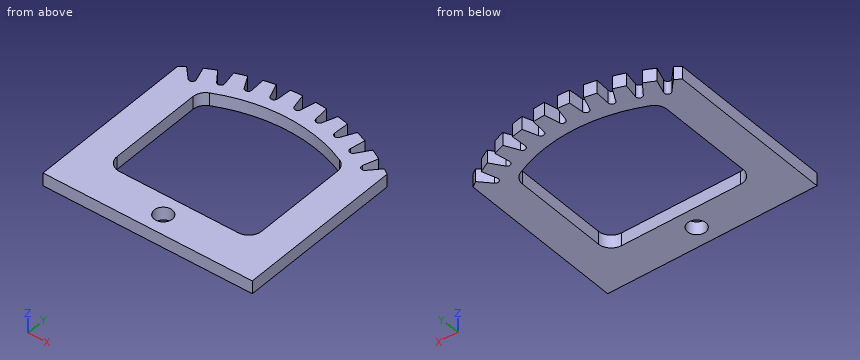
from build123d import *

# Parameters (mm, degrees)
ESQUISSE1_R        = 7
BOSS_EXTRU_2_DEPTH = 5


with BuildPart() as part:
    # Esquisse1 → Boss.-Extru.2 (new body, symmetric)
    with BuildSketch(Plane.XY):
        with BuildLine():
            Line((-81, 114.188440746), (-81, -15))
            Line((-81, -15), (81, -15))
            Line((81, -15), (81, 114.188440746))
            ThreePointArc((81, 114.188440746), (78.796472268, 115.719989449), (76.563994166, 117.209021825))
            Line((76.563994166, 117.209021825), (68.597490223, 108.845387152))
            ThreePointArc((68.597490223, 108.845387152), (65.420366542, 108.419035897), (64.316466092, 111.428569759))
            Line((64.316466092, 111.428569759), (68.001945903, 122.375387041))
            ThreePointArc((68.001945903, 122.375387041), (64.034003077, 124.497576081), (59.999908366, 126.491149872))
            Line((59.999908366, 126.491149872), (53.238382738, 117.126464015))
            ThreePointArc((53.238382738, 117.126464015), (50.148170341, 116.274127452), (48.64719318, 119.10661008))
            Line((48.64719318, 119.10661008), (50.81752925, 130.451442004))
            ThreePointArc((50.81752925, 130.451442004), (46.598920029, 132.017198319), (42.332170661, 133.446571058))
            Line((42.332170661, 133.446571058), (36.899996383, 123.253090169))
            ThreePointArc((36.899996383, 123.253090169), (33.953537336, 121.990446371), (32.083092779, 124.593776437))
            Line((32.083092779, 124.593776437), (32.698363453, 136.127943595))
            ThreePointArc((32.698363453, 136.127943595), (28.306685892, 137.10846631), (23.88576542, 137.947345789))
            Line((23.88576542, 137.947345789), (19.882863135, 127.112571065))
            ThreePointArc((19.882863135, 127.112571065), (17.134355274, 125.462845387), (14.928848702, 127.789136649))
            Line((14.928848702, 127.789136649), (13.977736553, 139.300476958))
            ThreePointArc((13.977736553, 139.300476958), (9.493772162, 139.677730115), (5, 139.910685796))
            Line((5, 139.910685796), (2.5, 128.633914537))
            ThreePointArc((2.5, 128.633914537), (0, 126.627452408), (-2.5, 128.633914537))
            Line((-2.5, 128.633914537), (-5, 139.910685796))
            ThreePointArc((-5, 139.910685796), (-9.493772162, 139.677730115), (-13.977736553, 139.300476958))
            Line((-13.977736553, 139.300476958), (-14.928848702, 127.789136649))
            ThreePointArc((-14.928848702, 127.789136649), (-17.134355274, 125.462845387), (-19.882863135, 127.112571065))
            Line((-19.882863135, 127.112571065), (-23.88576542, 137.947345789))
            ThreePointArc((-23.88576542, 137.947345789), (-28.306685892, 137.10846631), (-32.698363453, 136.127943595))
            Line((-32.698363453, 136.127943595), (-32.083092779, 124.593776437))
            ThreePointArc((-32.083092779, 124.593776437), (-33.953537336, 121.990446371), (-36.899996383, 123.253090169))
            Line((-36.899996383, 123.253090169), (-42.332170661, 133.446571058))
            ThreePointArc((-42.332170661, 133.446571058), (-46.598920029, 132.017198319), (-50.81752925, 130.451442004))
            Line((-50.81752925, 130.451442004), (-48.64719318, 119.10661008))
            ThreePointArc((-48.64719318, 119.10661008), (-50.148170341, 116.274127452), (-53.238382738, 117.126464015))
            Line((-53.238382738, 117.126464015), (-59.999908366, 126.491149872))
            ThreePointArc((-59.999908366, 126.491149872), (-64.034003077, 124.497576081), (-68.001945903, 122.375387041))
            Line((-68.001945903, 122.375387041), (-64.316466092, 111.428569759))
            ThreePointArc((-64.316466092, 111.428569759), (-65.420366542, 108.419035897), (-68.597490223, 108.845387152))
            Line((-68.597490223, 108.845387152), (-76.563994166, 117.209021825))
            ThreePointArc((-76.563994166, 117.209021825), (-78.796472268, 115.719989449), (-81, 114.188440746))
        make_face()
        Circle(ESQUISSE1_R, mode=Mode.SUBTRACT)
        with BuildLine():
            Line((-56, 97.713868002), (-56, 25))
            ThreePointArc((-56, 25), (-53.071067812, 17.928932188), (-46, 15))
            Line((-46, 15), (46, 15))
            ThreePointArc((46, 15), (53.071067812, 17.928932188), (56, 25))
            Line((56, 25), (56, 97.713868002))
            ThreePointArc((56, 97.713868002), (54.443713419, 103.071451759), (50.259259259, 106.761448373))
            ThreePointArc((50.259259259, 106.761448373), (0, 118), (-50.259259259, 106.761448373))
            ThreePointArc((-50.259259259, 106.761448373), (-54.443713419, 103.071451759), (-56, 97.713868002))
        make_face(mode=Mode.SUBTRACT)
    extrude(amount=BOSS_EXTRU_2_DEPTH, both=True)


solid = part.part
Verification items for the finished model (mm, model axes). Coordinates: 2 decimals unless noted, no trailing zeros. Order: outer loops, then holes, each group sorted by start corner. A loop starts at its lowest first (then second) coordinate and runs counter-clockwise, first axis right, second up. Notation, with made-up numbers: M 50,41 L 69,41 A27 cw 69,73 Z; hole C -28.5,57.25 d3. An arc over 180 degrees is marked long. Return JSON: item names as keys, results as strings.
1) Cross-section at A-A, the plane y = 70. Record the boundary of the cut face in (x, z), and give its area (3 significant figures).
Answer list:
{"outline": "M -81,-5 L -56,-5 L -56,5 L -81,5 Z; M 56,-5 L 81,-5 L 81,5 L 56,5 Z", "area": "500 mm2"}
2) Cross-section at D-D, the plane z = 0.5. Count the separate pieces of the cut face and the enclosed holes in it, and give its area (3 significant figures).
Answer list:
{"separate pieces": "1", "enclosed holes": "2", "area": "11,800 mm2"}
3) Gauge pin test, flat ends, axial feed: pin 1 (4 mm diameter, centred on x = -56.5, z = 3, fed in from +Y); pin 2 (11 mm diameter, centred on x = 0, y = 0, fed in from -Z); pin 3 (4 mm diameter, centred on x = 63.5, z = 2, fed in from +Y). Record the tip position at first contact, or that the pin passes through.
Answer list:
{"pin 1": "y = 124.41", "pin 2": "through", "pin 3": "y = 125.77"}
4) Cross-section at C-C, the plane x = 22. Record the boundary of the cut face in (y, z), and give its area (3 significant figures).
Answer list:
{"outline": "M -15,-5 L 15,-5 L 15,5 L -15,5 Z; M 115.93,-5 L 132.84,-5 L 132.84,5 L 115.93,5 Z", "area": "469 mm2"}
5) Cross-section at B-B, the plane x = 0. Record the boundary of the cut face in (y, z), and give its area (3 significant figures).
Answer list:
{"outline": "M -15,-5 L -7,-5 L -7,5 L -15,5 Z; M 7,-5 L 15,-5 L 15,5 L 7,5 Z; M 118,-5 L 126.63,-5 L 126.63,5 L 118,5 Z", "area": "246 mm2"}
6) Thickness scan on L1, parallel to Y at x = 0, z = 2.5; L2, parallel to X at y = 62.5, z = -0.5; L3, parallel to X at y = 105.5, z = -1.75. Record the ranges inside material, lowest first. Write a range as [from, to].
Answer list:
{"L1": "[-15, -7], [7, 15], [118, 126.63]", "L2": "[-81, -56], [56, 81]", "L3": "[-81, -52.28], [52.28, 81]"}
